Here's how the part is built. I have some questions about the finished solid (model axes, mm). Face numbers are marked on the shaded views. A direction names the side the tool comes from. Round coordinates to 2 decimals unless told otherwise and drop trailing zeros. Order: outer loops, then holes, each group sorted by start corner. A loop starts at its lowest first (then second) coordinate and runs counter-clockwise, first axis right, second up.
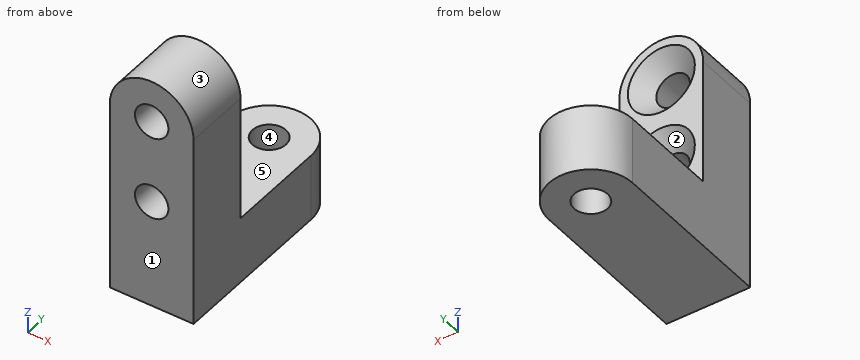
```python
from build123d import *

# Parameters (mm, degrees)
SKETCH_1_R      = 2
EXTRUDE_1_DEPTH = 8
SKETCH_2_R      = 2
EXTRUDE_2_DEPTH = 8
CHAMFER_1_SIZE  = 2


with BuildPart() as part:
    # 草图1 → 凸台-拉伸1 (new body)
    with BuildSketch(Plane.XY):
        with BuildLine():
            Line((-5, 20), (-5, 0))
            Line((-5, 0), (5, 0))
            Line((5, 0), (5, 20))
            ThreePointArc((5, 20), (0, 25), (-5, 20))
        make_face()
        with Locations((0, 20)):
            Circle(SKETCH_1_R, mode=Mode.SUBTRACT)
    extrude(amount=EXTRUDE_1_DEPTH)

    # 草图2 → 凸台-拉伸2 (add)
    with BuildSketch(Plane(origin=(0, 0, 0), x_dir=(1, 0, 0), z_dir=(0, 1, 0))):
        with BuildLine():
            Line((-5, -8), (5, -8))
            Line((5, -8), (5, -23))
            ThreePointArc((5, -23), (0, -28), (-5, -23))
            Line((-5, -23), (-5, -8))
        make_face()
        with Locations(Location((0, -23, 0), (0, 0, 270))):
            Circle(SKETCH_2_R, mode=Mode.SUBTRACT)
        with Locations(Location((0, -13, 0), (0, 0, 270))):
            Circle(SKETCH_2_R, mode=Mode.SUBTRACT)
    extrude(amount=EXTRUDE_2_DEPTH)

    # 倒角1
    chamfer_1_edges = [part.edges().sort_by_distance(p)[0] for p in [
        (0, 8, 21),
        (0, 8, 11),
    ]]
    chamfer(chamfer_1_edges, length=CHAMFER_1_SIZE)


solid = part.part
```
1) If we section it at C-C (y = 3.75): Write out the boundary of the cut face in (x, z), plus the area to 3 significant figures.
2) We'd pull the mould along X, two halves only. Please class the marked faces 1, 2 and 3: +X half, -X half, draft (parallel to the pull), parting line (faces both ways), or undercut.
3) I'm going to push flat-ended pins straight in: pin 1 (4 mm diameter, centred on x = -1, y = 18.5, fed in from +Z); pin 2 (6 mm diameter, centred on x = 2, z = 23.5, fed in from +Y). Where does each tip first touch, or does it pass through?
4) I need wall thicknesses on line 1 (Y direction, x = 0, z = 4.5); line 2 (X direction, y = 2.3, z = 23); line 3 (Y direction, x = -3.75, z = 17.5). Which ranges of each line are inside material? Lowest first, please.
5) If we section it at A-A (z = 13): Write out the boundary of the cut face in (x, y).
6) For the marked faces 4 and 5, which set-ups out of +Z, -Z, +X, -X, +Y, -Y let a thin tool reach every point of the face, with its end or its side?
7) If we section it at B-B (z = 2.5): Write out the boundary of the cut face in (x, y), plus the area to 3 significant figures.
8) If we section it at D-D (x = -0.5): Give the number of separate pieces and of enclosed holes in the cut face, plus the area to 3 significant figures.
Solutions:
1. outline: (-5, 0) - (5, 0) - (5, 23) arc R5 ccw to (-5, 23) - close; hole circle Ø4 at (0, 13); hole circle Ø4 at (0, 23)
1. area: 244 mm2
2. face 1: draft
2. face 2: undercut
2. face 3: parting line
3. pin 1: stops at z = 8
3. pin 2: stops at y = 8
4. line 1: y = 0 to 18, 22 to 25
4. line 2: x = -5 to -2, 2 to 5
4. line 3: y = 0 to 8
5. outline: (-5, 0) - (-2, 0) - (-2, 6) - (-4, 8) - (-5, 8) - close; (2, 0) - (5, 0) - (5, 8) - (4, 8) - (2, 6) - close
6. face 4: +Z, -Z
6. face 5: +Z, +X, -X, +Y
7. outline: (-5, 0) - (5, 0) - (5, 20) arc R5 ccw to (-5, 20) - close; hole circle Ø4 at (0, 20)
7. area: 227 mm2
8. separate pieces: 4
8. enclosed holes: 0
8. area: 258 mm2
